```python
from build123d import *

# Parameters (mm, degrees)
SKETCH1_W           = 85
SKETCH1_H           = 100
BOSS_EXTRUDE1_DEPTH = 45
SHELL1_T            = -2
SKETCH3_R           = 2.5
BOSS_EXTRUDE2_DEPTH = 3
SKETCH4_R           = 1.025
CUT_EXTRUDE1_DEPTH  = 2.7
SKETCH17_W          = 13.25
SKETCH17_H          = 16
SKETCH17_W_2        = 16
SKETCH17_H_2        = 13.5
CUT_EXTRUDE2_DEPTH  = 2
LPATTERN1_COUNT     = 2
LPATTERN1_PITCH     = 20
SKETCH18_R          = 1.7
CUT_EXTRUDE3_DEPTH  = 2
CUT_EXTRUDE9_DEPTH  = 10
CIRPATTERN2_COUNT   = 4
CIRPATTERN2_ANGLE   = 291
SKETCH19_4_W        = 4.949747468
SKETCH19_4_H        = 4.949747468
CUT_EXTRUDE10_DEPTH = 10


with BuildPart() as part:
    # Sketch1 → Boss-Extrude1 (new body)
    with BuildSketch(Plane(origin=(0, 0, 0), x_dir=(1, 0, 0), z_dir=(0, 1, 0))):
        Rectangle(SKETCH1_W, SKETCH1_H)
    extrude(amount=BOSS_EXTRUDE1_DEPTH)

    # Shell1
    shell1_openings = [part.faces().sort_by_distance(p)[0] for p in [
        (0, 0, 0),
    ]]
    offset(amount=SHELL1_T, openings=shell1_openings, kind=Kind.INTERSECTION)

    # Sketch3 → Boss-Extrude2 (add)
    with BuildSketch(Plane.XZ.offset(-43)):
        with Locations((-36.5, 24.5)):
            Circle(SKETCH3_R)
        with Locations((12.5, 24.5)):
            Circle(SKETCH3_R)
        with Locations((-36.5, -33.5)):
            Circle(SKETCH3_R)
        with Locations((12.5, -33.5)):
            Circle(SKETCH3_R)
    extrude(amount=BOSS_EXTRUDE2_DEPTH)

    # Sketch4 → Cut-Extrude1 (cut)
    with BuildSketch(Plane.XZ.offset(-40)):
        with Locations((12.5, 24.5)):
            Circle(SKETCH4_R)
        with Locations((-36.5, 24.5)):
            Circle(SKETCH4_R)
        with Locations((-36.5, -33.5)):
            Circle(SKETCH4_R)
        with Locations((12.5, -33.5)):
            Circle(SKETCH4_R)
    extrude(amount=-CUT_EXTRUDE1_DEPTH, mode=Mode.SUBTRACT)

    # Sketch17 → Cut-Extrude2 (cut)
    with BuildSketch(Plane.XY.offset(50)):
        with Locations((-31.065, 30.5)):
            Rectangle(SKETCH17_W, SKETCH17_H)
        with Locations((-13.065, 30.5)):
            Rectangle(SKETCH17_W, SKETCH17_H)
        with Locations((5.69, 31.75)):
            Rectangle(SKETCH17_W_2, SKETCH17_H_2)
    cut_extrude2 = extrude(amount=-CUT_EXTRUDE2_DEPTH, mode=Mode.SUBTRACT)

    # LPattern1: Cut-Extrude2 ×2
    with Locations(*[(0, -i * LPATTERN1_PITCH, 0) for i in range(1, LPATTERN1_COUNT)]):
        add(cut_extrude2, mode=Mode.SUBTRACT)

    # Sketch18 → Cut-Extrude3 (cut)
    with BuildSketch(Plane(origin=(42.5, 0, 0), x_dir=(0, 0, -1), z_dir=(1, 0, 0))):
        with Locations((15, 16)):
            Circle(SKETCH18_R)
        with Locations((-8.8, 16)):
            Circle(SKETCH18_R)
        with Locations((-8.8, 39.8)):
            Circle(SKETCH18_R)
        with Locations((15, 39.8)):
            Circle(SKETCH18_R)
    extrude(amount=-CUT_EXTRUDE3_DEPTH, mode=Mode.SUBTRACT)

    # Sketch19 → Cut-Extrude9 (cut)
    with BuildSketch(Plane(origin=(42.5, 0, 0), x_dir=(0, 0, -1), z_dir=(1, 0, 0))):
        Polygon((-6.364101615, 37.364101615), (-3.82820323, 27.9), (3.1, 34.82820323), align=None)
    cut_extrude9 = extrude(amount=-CUT_EXTRUDE9_DEPTH, mode=Mode.SUBTRACT)

    # CirPattern2: Cut-Extrude9 ×4 about axis
    cirpattern2_axis = Axis((0, 27.9, -3.1), (1, 0, 0))
    for i in range(1, CIRPATTERN2_COUNT):
        add(cut_extrude9.rotate(cirpattern2_axis, i * CIRPATTERN2_ANGLE / (CIRPATTERN2_COUNT - 1)), mode=Mode.SUBTRACT)

    # Sketch19<4> → Cut-Extrude10 (cut)
    with BuildSketch(Plane(origin=(42.5, 0, 0), x_dir=(0, 0, -1), z_dir=(1, 0, 0))):
        with Locations((3.1, 27.9)):
            Rectangle(SKETCH19_4_W, SKETCH19_4_H)
    extrude(amount=-CUT_EXTRUDE10_DEPTH, mode=Mode.SUBTRACT)


solid = part.part
```
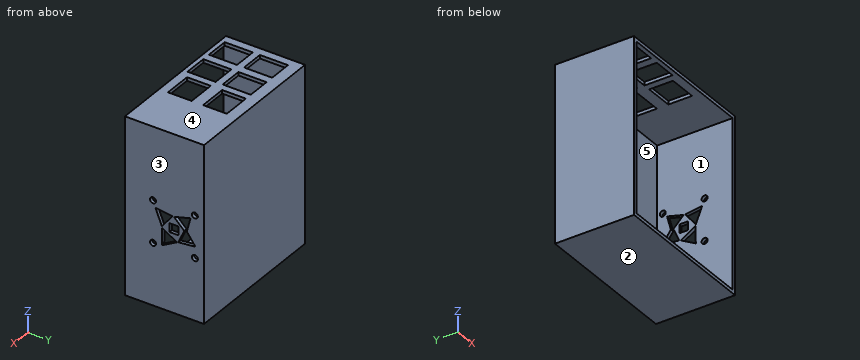
Input: part model. Units: mm. Frame: model coordinates. Face numbers are marked on the shaded views. A direction names the side the tool comes from. Give positions to 0.01 mm unless a question says otherwise; leave off trailing zeros. Order: outer loops, then holes, each group sorted by start corner. A loop starts at its lowest first (then second) coordinate and runs counter-clockwise, first axis right, second up. Notation, with made-up numbers: M 27,51.25 L 47,51.25 A22 cw 47,61.25 Z; hole C 58,35 d4. An arc over 180 degrees is marked long. Return JSON: item names as keys, results as strings.
Item 1: Cut plane A-A (y = 12). Return loops of the section in (x, z), then the cut area to 3 significant figures.
Solutions:
{"outline": "M -42.5,-50 L 42.5,-50 L 42.5,50 L 13.69,50 L 13.69,48 L 40.5,48 L 40.5,-48 L -40.5,-48 L -40.5,48 L -37.69,48 L -37.69,50 L -42.5,50 Z; M -24.44,48 L -19.69,48 L -19.69,50 L -24.44,50 Z; M -6.44,48 L -2.31,48 L -2.31,50 L -6.44,50 Z", "area": "639 mm^2"}
Item 2: First-contact query: P1, Ø6, axis at x = -28.5, z = -31, coming from the -Y side; P2, Ø2.5, axis at x = 13, z = -33, coming from the -Y side. Flat tips, straight axial feed; report the tip coordinate or a pass-through.
Solutions:
{"P1": "y = 43", "P2": "y = 40"}
Item 3: Ray query, probe 1 along Z at (x, y) = (-36.5, 41.6) (3 decimals); probe 2 along X at (y, z) = (13, -42); probe 3 along Z at (x, y) = (29.5, 7). Return the intervals inside material, ascending.
Solutions:
{"probe 1": "-50 to -48, -36 to -34.525, -32.475 to -31, 22 to 23.475, 25.525 to 27, 48 to 50", "probe 2": "-42.5 to -40.5, 40.5 to 42.5", "probe 3": "-50 to -48, 48 to 50"}
Item 4: Access query for the marked faces 1 and 2. Directions: +Z, -Z, +X, -X, +Y, -Y. A direction counts if a zero-diameter tool reaches every point of the face in a straight line with its end or side. Return the directions, or none.
Solutions:
{"face 1": "-Y", "face 2": "-Z, +X, -X, +Y, -Y"}
Item 5: Cut plane B-B (z = 38). Return loops of the section in (x, y).
Solutions:
{"outline": "M -42.5,0 L -40.5,0 L -40.5,43 L 40.5,43 L 40.5,0 L 42.5,0 L 42.5,45 L -42.5,45 Z"}
Item 6: Cut plane C-C (x = -21). Return loops of the section in (y, z).
Solutions:
{"outline": "M 0,-50 L 45,-50 L 45,50 L 0,50 L 0,48 L 43,48 L 43,-48 L 0,-48 Z"}
Item 7: Pull-direction query (Z, two-part tool) for the marked faces 3, 4 and 5; classes: +Z half, -Z half, draft (parallel to the pull), parting line (faces both ways), or undercut.
Solutions:
{"face 3": "draft", "face 4": "+Z half", "face 5": "undercut"}
